```python
from build123d import *

# Parameters (mm, degrees)
SKETCH2_W           = 374.6754
SKETCH2_H           = 254
BOSS_EXTRUDE2_DEPTH = 12.7
CUT_EXTRUDE1_DEPTH  = 453.834346495
FILLET1_R           = 7.62


with BuildPart() as part:
    # Sketch2 → Boss-Extrude2 (new body)
    with BuildSketch(Plane(origin=(0, 0, 0), x_dir=(1, 0, 0), z_dir=(0, 1, 0))):
        with Locations((187.3377, 127)):
            Rectangle(SKETCH2_W, SKETCH2_H)
    extrude(amount=BOSS_EXTRUDE2_DEPTH)

    # Sketch4 → Cut-Extrude1 (cut, through all)
    with BuildSketch(Plane(origin=(374.6754, 0, 0), x_dir=(0, 0, -1), z_dir=(1, 0, 0))):
        Polygon((101.961691264, 12.7), (0, 0), (0, 12.7), align=None)
    extrude(amount=-CUT_EXTRUDE1_DEPTH, mode=Mode.SUBTRACT)

    # Fillet1
    fillet1_edges = [part.edges().sort_by_distance(p)[0] for p in [
        (187.3377, 12.7, -101.961691264),
    ]]
    fillet(fillet1_edges, radius=FILLET1_R)


solid = part.part
```
Here's how the part is built. I have some questions about the finished solid (model axes, mm). Round coordinates to 2 decimals unless told otherwise and drop trailing zeros. Order: outer loops, then holes, each group sorted by start corner. A loop starts at its lowest first (then second) coordinate and runs counter-clockwise, first axis right, second up. Notation, with made-up numbers: (-40, 79.25) -> (-26, 79.25) arc R34 cw to (-26, 117.25) -> close; hole circle Ø11 at (-26.75, -15.75). An arc over 180 degrees is marked (long way). Use a Markdown table: item, result. Add a question column.
(1) Suppose I cut it at A-A, the plane x = 83. Please give me the cut outline in (y, z).
(2) Suppose I cut it at B-B, the plane z = -94. Please give me the cut outline in (x, y).
(3) I need wall thicknesses on line 1 along Y through (x, z) = (52.5, -89). Which ranges of the line are inside material? Lowest first, please.
(4) Suppose I cut it at C-C, the plane y = 5.75. Please give me the cut outline in (x, z).
(5) For pin 1 Ø3 at (x, z) = (289.5, -96.5) entering from +Y, with a flat end and sliding along its axis, tell me the tip position at first contact or that it passes through.
Verdict:
| question | item | result |
|---|---|---|
| 1 | outline | (0, -254) -> (12.7, -254) -> (12.7, -102.43) arc R7.62 ccw to (12.64, -101.49) -> (0, 0) -> close |
| 2 | outline | (0, 0) -> (374.68, 0) -> (374.68, 11.71) -> (0, 11.71) -> close |
| 3 | line 1 | 0 to 11.09 |
| 4 | outline | (0, -254) -> (374.68, -254) -> (374.68, -46.16) -> (0, -46.16) -> close |
| 5 | pin 1 | y = 12.21 |
